Could you check a few things on this model? Use its own coordinates, in mm. A direction names the side the tool comes from. Round coordinates to 2 decimals unless told otherwise and drop trailing zeros. Loops run counter-clockwise (first coordinate to the right, second up) from the corner with the lowest first, then second, coordinate; pieces in that order, holes last. Notation, with made-up numbers: (-25, 28) -> (5, 28) arc R16 ccw to (5, 56) -> close; hole circle Ø7 at (-25, 81). An arc over 180 degrees is marked (long way). One line per item, written item: value.
```python
from build123d import *

# Parameters (mm, degrees)
SKETCH1_W            = 203.2
SKETCH1_H            = 127
BOSS_EXTRUDE1_DEPTH  = 6.35
M3_CLEARANCE_HOLE1_D = 3.4
SKETCH6_W            = 101.6
SKETCH6_H            = 76.2
CUT_EXTRUDE3_DEPTH   = 240.70724332
FILLET1_R            = 6.35


with BuildPart() as part:
    # Sketch1 → Boss-Extrude1 (new body)
    with BuildSketch(Plane.XY):
        with Locations((101.6, 63.5)):
            Rectangle(SKETCH1_W, SKETCH1_H)
    extrude(amount=BOSS_EXTRUDE1_DEPTH)

    # M3 Clearance Hole1 (through all)
    with Locations(Plane.XY.offset(6.35)):
        with Locations((5.9944, 121.0056), (5.9944, 21.9964), (197.2056, 21.9964), (197.2056, 121.0056)):
            Hole(M3_CLEARANCE_HOLE1_D / 2)

    # Sketch6 → Cut-Extrude3 (cut, through all)
    with BuildSketch(Plane.XY.offset(6.35)):
        with Locations((101.6, 63.5)):
            Rectangle(SKETCH6_W, SKETCH6_H)
    extrude(amount=-CUT_EXTRUDE3_DEPTH, mode=Mode.SUBTRACT)

    # Fillet1
    fillet1_edges = [part.edges().sort_by_distance(p)[0] for p in [
        (152.4, 101.6, 3.175),
        (152.4, 25.4, 3.175),
        (50.8, 25.4, 3.175),
        (50.8, 101.6, 3.175),
    ]]
    fillet(fillet1_edges, radius=FILLET1_R)


solid = part.part
```
(1) Imagine slicing it at C-C on z = 2.75. Write out the boundary of the cut face in (x, y).
Results below:
outline: (0, 0) -> (203.2, 0) -> (203.2, 127) -> (0, 127) -> close; hole circle Ø3.4 at (5.99, 22); hole circle Ø3.4 at (5.99, 121.01); hole (50.8, 31.75) arc R6.35 ccw to (57.15, 25.4) -> (146.05, 25.4) arc R6.35 ccw to (152.4, 31.75) -> (152.4, 95.25) arc R6.35 ccw to (146.05, 101.6) -> (57.15, 101.6) arc R6.35 ccw to (50.8, 95.25) -> close; hole circle Ø3.4 at (197.21, 22); hole circle Ø3.4 at (197.21, 121.01)
(2) Please list where these lines run through material, in increasing order: L1, parallel to X at y = 41, z = 2.25; L2, parallel to Y at x = 63.5, z = 1.75; L3, parallel to Y at x = 148, z = 0.75.
Results below:
L1: x = 0 to 50.8, 152.4 to 203.2
L2: y = 0 to 25.4, 101.6 to 127
L3: y = 0 to 25.71, 101.29 to 127
(3) Imagine slicing it at A-A on y = 89. Write out the boundary of the cut face in (x, z).
Results below:
outline: (0, 0) -> (50.8, 0) -> (50.8, 6.35) -> (0, 6.35) -> close; (152.4, 0) -> (203.2, 0) -> (203.2, 6.35) -> (152.4, 6.35) -> close
(4) On a 3-axis mill with a long thin cutter (end or side, diameter ignored), from which of +Z, -Z, +X, -X, +Y, -Y can I reach the whole of each face in a straight line? I mean faces 1 (the face through (0, 63, 3)), 2 (the face through (101, 101.6, 3)). Say none if no direction works.
Results below:
face 1: +Z, -Z, -X, +Y, -Y
face 2: +Z, -Z
(5) We'd pull the mould along X, two halves only. Please class faces 3 (the face through (203.2, 63, 3)), 4 (the face through (100, 22, 6.35)), 5 (the face through (52.71, 99.79, 3.13)): +X half, -X half, draft (parallel to the pull), parting line (faces both ways), or undercut.
Results below:
face 3: +X half
face 4: draft
face 5: undercut
(6) Imagine slicing it at B-B on x = 62.5. Write out the boundary of the cut face in (y, z), then the cut area to 3 significant figures.
Results below:
outline: (0, 0) -> (25.4, 0) -> (25.4, 6.35) -> (0, 6.35) -> close; (101.6, 0) -> (127, 0) -> (127, 6.35) -> (101.6, 6.35) -> close
area: 323 mm²
